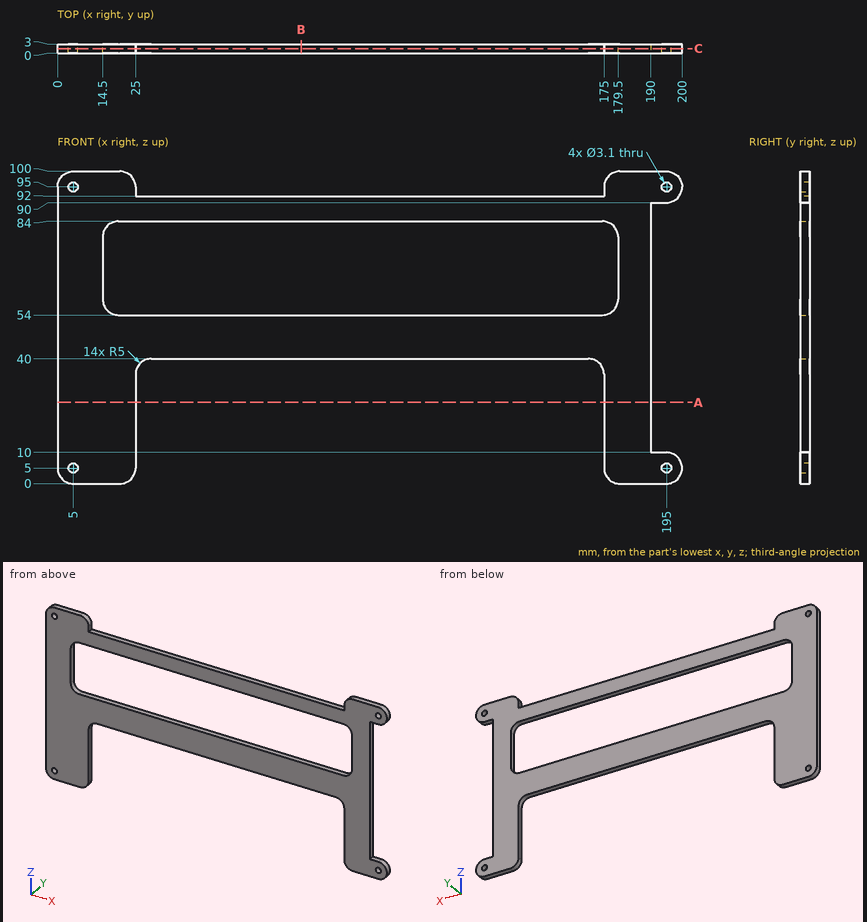
Design review of the part shown in the three views and the two pictorial views. Dimensions are in mm from the part's minimum x, y and z. Give positions to 0.01 mm unless a question says otherwise; leave off trailing zeros. Loops run counter-clockwise (first coordinate to the right, second up) from the corner with the lowest first, then second, coordinate; pieces in that order, holes last. Notation, with made-up numbers: (-21.5, -11.5) -> (6.5, -11.5) arc R12 ccw to (6.5, 1.5) -> close; hole circle Ø2 at (-7.75, -34). An arc over 180 degrees is marked (long way). Write each question's results on one line, items separated by ' | '.
1) Take a section at A-A, the plane z = 26. Give the boundary of the cut face in (x, y).
Conclusion:
outline: (0, 0) -> (25, 0) -> (25, 3) -> (0, 3) -> close; (175, 0) -> (190, 0) -> (190, 3) -> (175, 3) -> close
2) Take a section at C-C, the plane y = 1.5. Count the separate pieces of the cut face and the enclosed holes in it, plus the area to 3 significant figures.
Conclusion:
separate pieces: 1 | enclosed holes: 5 | area: 7,000 mm^2
3) For line 1 along X through (y, z) = (2.3, 5); line 2 along Z through (x, y) = (5, 1.2); line 3 along Z through (x, y) = (195, 1.2), list the stretches that pass through material, from the lowest coordinate up. Write a range as from..to.
Conclusion:
line 1: x = 0..3.45, 6.55..25, 175..193.45, 196.55..200 | line 2: z = 0..3.45, 6.55..93.45, 96.55..100 | line 3: z = 0..3.45, 6.55..10, 90..93.45, 96.55..100
4) Insertion check: pin 1 Ø1.5 at (y, z) = (2, 16) entering from +X; pin 2 Ø0.9 at (x, y) = (127.5, 1) entering from -Z. Each pin has a flat end and moves straight along its axis. Give the tip position at first contact, or say it passes through.
Conclusion:
pin 1: stops at x = 190 | pin 2: stops at z = 40
5) Take a section at B-B, the plane x = 78. Give the boundary of the cut face in (y, z), plus the area to 3 significant figures.
Conclusion:
outline: (0, 40) -> (3, 40) -> (3, 54) -> (0, 54) -> close; (0, 84) -> (3, 84) -> (3, 92) -> (0, 92) -> close | area: 66.0 mm^2
